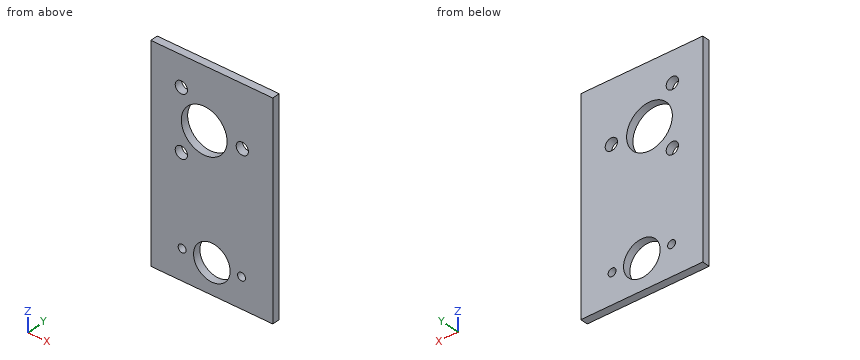
from build123d import *

# Parameters (mm, degrees)
SKETCH1_W           = 50.8
SKETCH1_H           = 88.138
BOSS_EXTRUDE1_DEPTH = 3.175
SKETCH2_R           = 2.5527
SKETCH2_R_2         = 9.525
CUT_EXTRUDE1_DEPTH  = 3.175
SKETCH4_R           = 1.651
SKETCH4_R_2         = 7.62
CUT_EXTRUDE2_DEPTH  = 3.175


with BuildPart() as part:
    # Sketch1 → Boss-Extrude1 (new body)
    with BuildSketch(Plane(origin=(0, 0, 0), x_dir=(1, 0, 0), z_dir=(0, 1, 0))):
        with Locations((25.4, 44.069)):
            Rectangle(SKETCH1_W, SKETCH1_H)
    extrude(amount=BOSS_EXTRUDE1_DEPTH)

    # Sketch2 → Cut-Extrude1 (cut)
    with BuildSketch(Plane(origin=(0, 3.175, 0), x_dir=(1, 0, 0), z_dir=(0, 1, 0))):
        with Locations((12.7, 12.7)):
            Circle(SKETCH2_R)
        with Locations((12.7, 38.1)):
            Circle(SKETCH2_R)
        with Locations((38.1, 25.4)):
            Circle(SKETCH2_R)
        with Locations((22.225, 25.4)):
            Circle(SKETCH2_R_2)
    extrude(amount=-CUT_EXTRUDE1_DEPTH, mode=Mode.SUBTRACT)

    # Sketch4 → Cut-Extrude2 (cut)
    with BuildSketch(Plane(origin=(0, 3.175, 0), x_dir=(1, 0, 0), z_dir=(0, 1, 0))):
        with Locations((13.0175, 75.438)):
            Circle(SKETCH4_R)
        with Locations((37.7825, 75.438)):
            Circle(SKETCH4_R)
        with Locations((25.4, 75.438)):
            Circle(SKETCH4_R_2)
    extrude(amount=-CUT_EXTRUDE2_DEPTH, mode=Mode.SUBTRACT)


solid = part.part
Work out the finished part from the listing and answer in its coordinate system (mm). Give positions to 0.01 mm unless a question says otherwise; leave off trailing zeros. Order: outer loops, then holes, each group sorted by start corner. A loop starts at its lowest first (then second) coordinate and runs counter-clockwise, first axis right, second up. Notation, with made-up numbers: M -29.5,15 L 8.5,15 A13 cw 8.5,33 Z; hole C 15.5,69 d4. An arc over 180 degrees is marked long. Return JSON: item names as keys, results as strings.
Q1. Find section B-B, the plane z = -12.7. Write down the section's boundary in (x, y) (3 decimals).
Answer below:
{"outline": "M 0,0 L 10.147,0 L 10.147,3.175 L 0,3.175 Z; M 15.253,0 L 50.8,0 L 50.8,3.175 L 15.253,3.175 Z"}
Q2. Find section A-A, the plane z = -25.4. Write down the section's boundary in (x, y) (3 decimals), and give its area (3 significant figures).
Answer below:
{"outline": "M 0,0 L 12.7,0 L 12.7,3.175 L 0,3.175 Z; M 31.75,0 L 35.547,0 L 35.547,3.175 L 31.75,3.175 Z; M 40.653,0 L 50.8,0 L 50.8,3.175 L 40.653,3.175 Z", "area": "84.6 mm^2"}
Q3. This flat-tipped pin is pushed along its axis until it touches: pin 1 (2 mm diameter, centred on x = 42.5, z = -29.5, fed in from -Y). Where does it stop, or does it pass through?
Answer below:
{"pin 1": "stops at y = 0"}
Q4. Find section D-D, the plane y = 2.4. State how many separate pieces and enclosed holes the cut face has, and give its area (3 significant figures).
Answer below:
{"separate pieces": "1", "enclosed holes": "7", "area": "3,930 mm^2"}
Q5. Find section C-C, the plane x = 20. Write down the section's boundary in (y, z) (3 decimals).
Answer below:
{"outline": "M 0,-88.138 L 3.175,-88.138 L 3.175,-80.814 L 0,-80.814 Z; M 0,-70.062 L 3.175,-70.062 L 3.175,-34.661 L 0,-34.661 Z; M 0,-16.139 L 3.175,-16.139 L 3.175,0 L 0,0 Z"}
Q6. Find the intervals of material crossed by line 1 along Z through (x, y) = (38, 1.1); line 2 along Z through (x, y) = (30, 1.5); line 3 along X through (y, z) = (1.55, -23.5), in increasing order. Write a range as [from, to].
Answer below:
{"line 1": "z = [-88.14, -77.07], [-73.8, -27.95], [-22.85, 0]", "line 2": "z = [-88.14, -81.51], [-69.36, -30.9], [-19.9, 0]", "line 3": "x = [0, 12.89], [31.56, 36.4], [39.8, 50.8]"}
